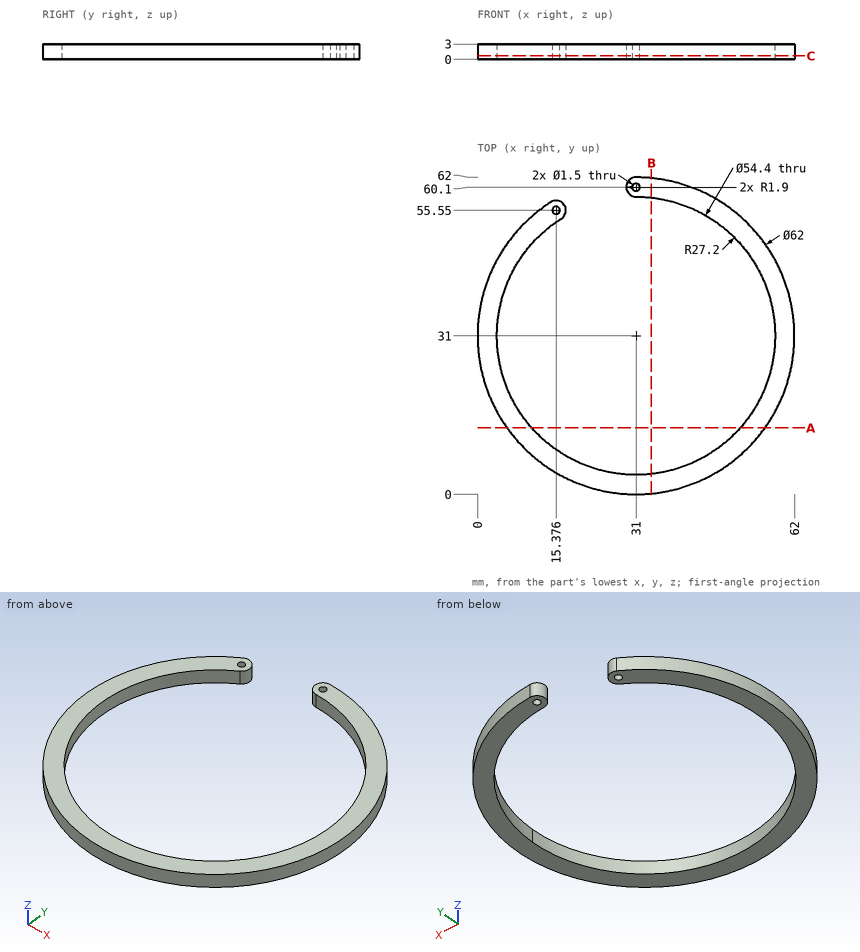
Input: dimensioned drawing with shaded views. Units: mm. Origin: part minimum x, y, z. Give positions to 0.01 mm unless a question says otherwise; leave off trailing zeros. Write each loop counter-clockwise with the first axis right and the second up, starting at its lowest first coordinate (ties: lowest second). Pieces come first, ordered by that corner, then holes.
1. Material intervals for line 1 along X through (y, z) = (31, 2.25); line 2 along X through (y, z) = (19.5, 1.45); line 3 along Y through (x, z) = (45, 2.7), sorted ascending.
2. First-contact query: pin 1 (1.4 mm diameter, centred on x = 31, y = 60.1, fed in from -Z); pin 2 (1 mm diameter, centred on y = 46.5, z = 2.5, fed in from -X); pin 3 (12 mm diameter, centred on x = 8, y = 23.5, fed in from +Z). Flat tips, straight axial feed; report the tip coordinate or a pass-through.
3. Section query C-C (z = 0.7). Return the cut outline in (x, y).
4. Section query B-B (x = 34). Return the cut outline in (y, z) (1 decimal), then the cut area to 3 significant figures.
5. Section query A-A (y = 13). Return the cut outline in (x, z).
Output values:
1. line 1: x = 0 to 3.8, 58.2 to 62
1. line 2: x = 2.21 to 6.35, 55.65 to 59.79
1. line 3: y = 3.34 to 7.68, 54.32 to 58.66
2. pin 1: passes through
2. pin 2: stops at x = 3.87
2. pin 3: stops at z = 3
3. outline: (14.36, 57.15) arc R31 ccw (long way) to (31, 62) arc R1.9 ccw to (31, 58.2) arc R27.2 cw (long way) to (16.4, 53.95) arc R1.9 ccw to start; hole circle Ø1.5 at (15.38, 55.55); hole circle Ø1.5 at (31, 60.1)
4. outline: (0.1, 0) - (4, 0) - (4, 3) - (0.1, 3) - close; (58, 0) - (61.9, 0) - (61.9, 3) - (58, 3) - close
4. area: 22.9 mm2
5. outline: (5.76, 0) - (10.61, 0) - (10.61, 3) - (5.76, 3) - close; (51.39, 0) - (56.24, 0) - (56.24, 3) - (51.39, 3) - close
